from build123d import *

# Parameters (mm, degrees)
F1_DEPTH = 25.4
F2_W     = 42.545
F2_H     = 3.057748
F3_DEPTH = 12.7
F4_R     = 1.27


with BuildPart() as f1:
    # F0 (on Front) → F1 (new body)
    with BuildSketch(Plane.XZ):
        with BuildLine():
            Line((42.545, 0), (0, 0))
            Line((0, 0), (0, -1.5875))
            Line((0, -1.5875), (42.622831, -1.5875))
            ThreePointArc((42.622831, -1.5875), (44.12669, -1.039864), (44.92625, 0.346572))
            Line((44.92625, 0.346572), (48.10125, 0.346572))
            ThreePointArc((48.10125, 0.346572), (48.90081, -1.039864), (50.404669, -1.5875))
            ThreePointArc((50.404669, -1.5875), (51.908529, -1.039864), (52.708089, 0.346572))
            Line((52.708089, 0.346572), (55.883089, 0.346572))
            ThreePointArc((55.883089, 0.346572), (56.682648, -1.039864), (58.186508, -1.5875))
            ThreePointArc((58.186508, -1.5875), (59.690368, -1.039864), (60.489927, 0.346572))
            Line((60.489927, 0.346572), (63.664927, 0.346572))
            ThreePointArc((63.664927, 0.346572), (64.464487, -1.039864), (65.968346, -1.5875))
            ThreePointArc((65.968346, -1.5875), (67.472206, -1.039864), (68.271766, 0.346572))
            Line((68.271766, 0.346572), (73.691467, 0.346572))
            Line((73.691467, 0.346572), (73.691467, 1.5875))
            Line((73.691467, 1.5875), (67.341467, 1.5875))
            ThreePointArc((67.341467, 1.5875), (65.833294, 0.495549), (64.32512, 1.5875))
            Line((64.32512, 1.5875), (59.56262, 1.5875))
            ThreePointArc((59.56262, 1.5875), (58.119729, 0.661984), (56.676839, 1.5875))
            Line((56.676839, 1.5875), (51.914339, 1.5875))
            ThreePointArc((51.914339, 1.5875), (50.404669, 0.490973), (48.895, 1.5875))
            Line((48.895, 1.5875), (44.1325, 1.5875))
            add(Edge.make_bspline(
                [(42.545, 0), (43.173972, 0), (43.24261, 0.79375), (43.695807, 1.5875), (44.1325, 1.5875)],
                knots=[0, 0, 0, 0, 1.122532, 2.245064, 2.245064, 2.245064, 2.245064], degree=3))
        make_face()
    extrude(amount=F1_DEPTH)

    # F2 (on face) → F3 (cut, symmetric)
    with BuildSketch(Plane.XY):
        with Locations((21.2725, -1.528874)):
            Rectangle(F2_W, F2_H)
        with BuildLine():
            Line((42.545, 0), (42.545, -3.057748))
            ThreePointArc((42.545, -3.057748), (58.193101, -2.291478), (73.691467, 0))
            Line((73.691467, 0), (42.545, 0))
        make_face()
        with Locations((21.2725, -23.871126)):
            Rectangle(F2_W, F2_H)
        with BuildLine():
            ThreePointArc((73.691467, -25.4), (58.193101, -23.108522), (42.545, -22.342252))
            Line((42.545, -22.342252), (42.545, -25.4))
            Line((42.545, -25.4), (73.691467, -25.4))
        make_face()
    extrude(amount=F3_DEPTH, both=True, mode=Mode.SUBTRACT)

    # F4
    f4_edges = [f1.edges().sort_by_distance(p)[0] for p in [
        (48.895, -12.7, 1.5875),
        (44.1325, -12.7, 1.5875),
        (51.914339, -12.7, 1.5875),
        (56.676839, -12.7, 1.5875),
        (59.56262, -12.7, 1.5875),
        (64.32512, -12.7, 1.5875),
        (67.341467, -12.7, 1.5875),
    ]]
    fillet(f4_edges, radius=F4_R)


solid = f1.part
CAD build for the part. Positions are in the model's coordinates, mm. A direction names the side the tool comes from. Round coordinates to 2 decimals unless told otherwise and drop trailing zeros. Order: outer loops, then holes, each group sorted by start corner. A loop starts at its lowest first (then second) coordinate and runs counter-clockwise, first axis right, second up. Notation, with made-up numbers: (55.5, 34.5) -> (107.5, 34.5) arc R19 cw to (107.5, 67.5) -> close; hole circle Ø1 at (-26.5, 30.25). An arc over 180 degrees is marked (long way). Write item = value, one per line. Start each with the question number.
(1) Pull direction X, two halves, no side cores. Call faces 1 (the cylindrical face through (58.138, -12.553, 0.662)), 2 (the cylindrical face through (58.41, -23.13, 0.38)), 3 (the flat face through (21, -22.342, -1)): released by +X, released by -X, zero draft, split by the parting line, or undercut.
(2) Probe line 1 (X direction, y = -21, z = -1.4); line 2 (X direction, y = -13.75, z = 0.25); line 3 (Z direction, x = 54.5, y = -13.5). List the from-to ranges inside material, lowest first. Write a range as [from, to].
(3) Which spindle directions (+Z, -Z, +X, -X, +Y, -Y) get a long thin tool onto all of the face, cutting with end or side? Do faces 4 (the flat face through (22, -13, 0)), 5 (the flat face through (71, -13, 0.347)), 6 (the flat face through (21, -3.058, -1)), 7 (the flat face through (62, -13, 0.347)). Say none if no direction does.
(4) Cut at B-B, the plane x = 53.5. List the corners of the cut face in (y, z).
(5) Cut at A-A, the plane x = 38. List the corners of the cut face in (y, z).
(6) Pin check, flat tips, straight feed: P1, Ø1, axis at y = -20, z = 0, coming from the -X side; P2, Ø0.5, axis at x = 28.5, z = -1, coming from the +Y side; P3, Ø3.5, axis at x = 62, y = -15.5, coming from the -Z side; P4, Ø12, axis at x = 30, y = -12, coming from the +Z side. Stop position of each tip, or through.
Model answer:
q1.face_1 = undercut
q1.face_2 = released by -X
q1.face_3 = zero draft
q2.line_1 = [0, 43.54], [49.49, 51.32], [57.27, 59.1], [65.05, 66.89]
q2.line_2 = [43.13, 44.91], [48.12, 52.69], [55.9, 60.47], [63.68, 68.25]
q2.line_3 = [0.35, 1.59]
q3.face_4 = +Z, -X, +Y, -Y
q3.face_5 = -Z, +X, +Y, -Y
q3.face_6 = +Z, -Z, -X, +Y
q3.face_7 = -Z, +Y, -Y
q4.outline = (-22.72, 0.35) -> (-2.68, 0.35) -> (-2.68, 1.59) -> (-22.72, 1.59) -> close
q5.outline = (-22.34, -1.59) -> (-3.06, -1.59) -> (-3.06, 0) -> (-22.34, 0) -> close
q6.P1 = 0
q6.P2 = -3.06
q6.P3 = -0.35
q6.P4 = 0
